Model file for the job. Use its own axes, mm. A direction names the side the tool comes from. Give positions to 0.01 mm unless a question says otherwise; leave off trailing zeros. Write each loop counter-clockwise with the first axis right and the second up, starting at its lowest first coordinate (ties: lowest second). Pieces come first, ordered by that corner, then holes.
```python
from build123d import *

# Parameters (mm, degrees)
BOSS_EXTRUDE1_DEPTH = 15.875
SKETCH6_R           = 7.9121
BOSS_EXTRUDE2_DEPTH = 50.8
CHAMFER1_SIZE       = 1.27
CHAMFER1_SIZE2      = 0.733234842


with BuildPart() as part:
    # Sketch1 → Boss-Extrude1 (new body)
    with BuildSketch(Plane(origin=(0, 0, 0), x_dir=(1, 0, 0), z_dir=(0, 1, 0))):
        Polygon((0, -15.58124039), (13.49375, -7.790620195), (13.49375, 7.790620195), (0, 15.58124039), (-13.49375, 7.790620195), (-13.49375, -7.790620195), align=None)
    extrude(amount=BOSS_EXTRUDE1_DEPTH)

    # Sketch2 → Cut-Revolve1 (revolve, cut)
    with BuildSketch(Plane(origin=(0, 0, 0), x_dir=(0, 0, -1), z_dir=(1, 0, 0))):
        with BuildLine():
            Line((13.54924039, 15.875), (15.58124039, 15.875))
            Line((15.58124039, 15.875), (15.58124039, 13.843))
            ThreePointArc((15.58124039, 13.843), (14.986081369, 15.279840979), (13.54924039, 15.875))
        make_face()
    revolve(axis=Axis((0, 15.875, 0), (0, -1, 0)), mode=Mode.SUBTRACT)

    # Sketch6 → Boss-Extrude2 (add)
    with BuildSketch(Plane.XZ):
        Circle(SKETCH6_R)
    extrude(amount=BOSS_EXTRUDE2_DEPTH)

    # Chamfer1
    chamfer1_edges = [part.edges().sort_by_distance(p)[0] for p in [
        (-7.9121, -50.8, 0),
    ]]
    chamfer1_side = [part.faces().sort_by_distance(p)[0] for p in [
        (-7.9121, -25.4, 0),
    ]]
    chamfer(chamfer1_edges, length=CHAMFER1_SIZE, length2=CHAMFER1_SIZE2, reference=chamfer1_side[0])


solid = part.part
```
1. Which spindle directions (+Z, -Z, +X, -X, +Y, -Y) get a long thin tool onto all of the face, cutting with end or side? Do faces 1 (the cylindrical face through (-1.715, -24.418, -7.724)), 2 (the flat face through (6.84, 7.83, -11.63)). Say none if no direction does.
Calculated:
face 1: -Y
face 2: -Z, +X, +Y, -Y
2. Slice it at A-A, the plane z = 0. Write the cut outline in (x, y) (3 decimals), and give its area (3 significant figures).
Calculated:
outline: (-13.494, 0) - (-7.912, 0) - (-7.912, -49.53) - (-7.179, -50.8) - (7.179, -50.8) - (7.912, -49.53) - (7.912, 0) - (13.494, 0) - (13.494, 15.875) - (-13.494, 15.875) - close
area: 1,230 mm2
3. Slice it at C-C, the plane y = -18.5. Write the cut outline in (x, z).
Calculated:
outline: circle Ø15.82 at (0, 0)
4. Slice it at B-B, the plane y = 11.5. Write the cut outline in (x, z).
Calculated:
outline: (-13.49, -7.79) - (0, -15.58) - (13.49, -7.79) - (13.49, 7.79) - (0, 15.58) - (-13.49, 7.79) - close
5. Pin check, flat tips, straight feed: P1, Ø8, axis at x = 3.5, z = 7, coming from the -Y side; P2, Ø3, axis at x = -6.5, y = -12, coming from the -Z side; P3, Ø1, axis at x = 5.5, z = 10, coming from the -Y side; P4, Ø1, axis at x = -6.5, y = -21, coming from the +Z side. Stop position of each tip, or through.
Calculated:
P1: stops at y = -50.8
P2: stops at z = -6.13
P3: stops at y = 0
P4: stops at z = 5.16
6. Probe probe 1 along Y at (x, z) = (-11, 3) (3 decimals); probe 2 along Z at (x, y) = (0, -39.5); probe 3 along X at (y, z) = (-6, 1). List the from-to ranges inside material, lowest first.
Calculated:
probe 1: y = 0 to 15.875
probe 2: z = -7.91 to 7.91
probe 3: x = -7.85 to 7.85
